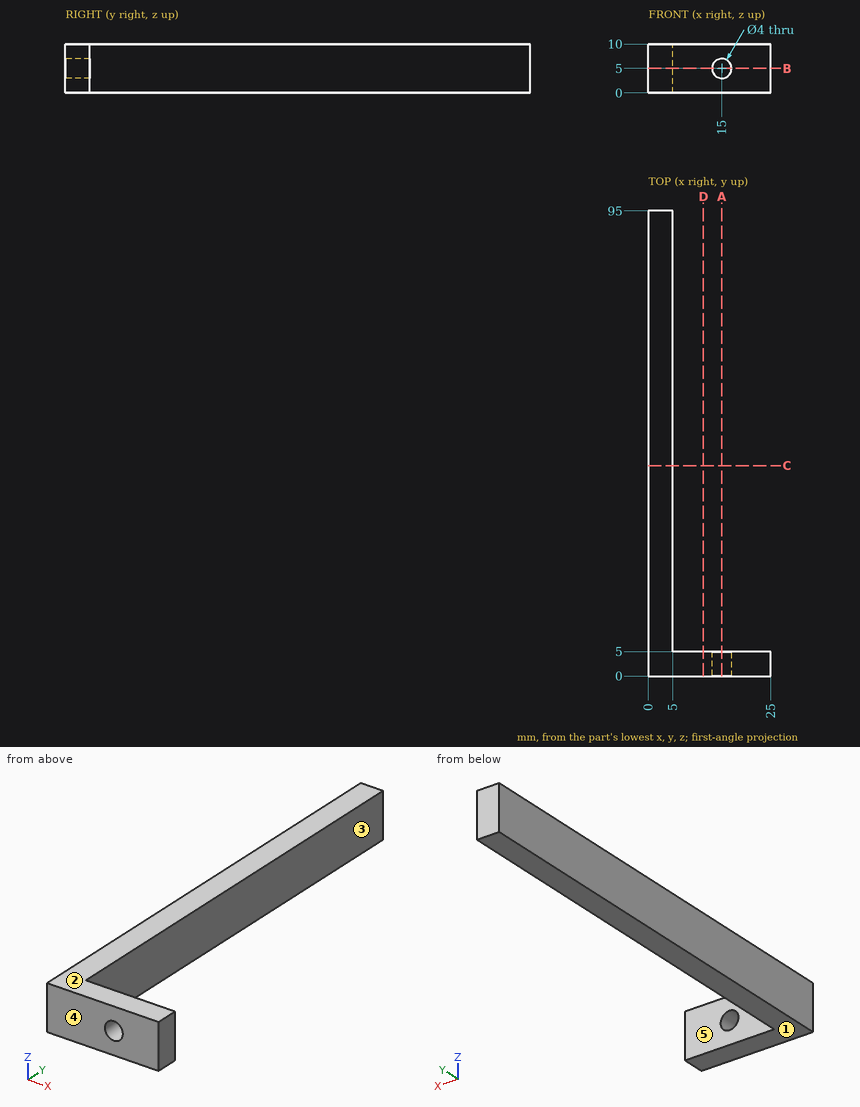
Part print with two shaded views. Sizes in mm from the minimum x, y, z corner. A direction names the side the tool comes from. Round coordinates to 2 decimals unless told otherwise and drop trailing zeros. Order: outer loops, then holes, each group sorted by start corner. A loop starts at its lowest first (then second) coordinate and runs counter-clockwise, first axis right, second up. Notation, with made-up numbers: (58.5, -16.75) - (110.5, -16.75) arc R16 cw to (110.5, -9.75) - close; hole circle Ø7 at (53.5, -8). An arc over 180 degrees is marked (long way). Answer in a Markdown table with one row per item. Add a question column.
(1) 3-axis set-ups, long thin cutter, end or side, ignore diameter. For the marked faces 4 and 5: which of +Z, -Z, +X, -X, +Y, -Y reach the whole face in a straight line?
(2) Drop flat-ended pins along their axis: pin 1 Ø4 at (y, z) = (35.5, 4.5) entering from +X; pin 2 Ø1.5 at (x, z) = (17, 2.5) entering from +Y. Give the stop position or say it passes through.
(3) Mould opens along Z. For the marked faces 1, 2 and 3 say: +Z half, -Z half, draft (parallel to the pull), parting line (faces both ways), or undercut.
(4) Band-saw the part on C-C on y = 43. List the corners of the cut face in (x, z).
(5) Probe L1, parallel to Z at x = 15, y = 3.2; L2, parallel to X at y = 49, z = 3.5. List the from-to ranges inside material, lowest first. Write a range as [from, to].
(6) Band-saw the part on B-B on z = 5. List the corners of the cut face in (x, y).
(7) Band-saw the part on A-A on x = 15. List the corners of the cut face in (y, z).
Data:
| question | item | result |
|---|---|---|
| 1 | face 4 | +Z, -Z, +X, -X, -Y |
| 1 | face 5 | +Z, -Z, +X, +Y |
| 2 | pin 1 | stops at x = 5 |
| 2 | pin 2 | stops at y = 5 |
| 3 | face 1 | -Z half |
| 3 | face 2 | +Z half |
| 3 | face 3 | draft |
| 4 | outline | (0, 0) - (5, 0) - (5, 10) - (0, 10) - close |
| 5 | L1 | z = [0, 3], [7, 10] |
| 5 | L2 | x = [0, 5] |
| 6 | outline | (0, 0) - (13, 0) - (13, 5) - (5, 5) - (5, 95) - (0, 95) - close; (17, 0) - (25, 0) - (25, 5) - (17, 5) - close |
| 7 | outline | (0, 0) - (5, 0) - (5, 3) - (0, 3) - close; (0, 7) - (5, 7) - (5, 10) - (0, 10) - close |
